Geometry check sheet. Reference: drawing and pictorial views, mm from the part's lowest x, y, z. A direction names the side the tool comes from. Round coordinates to 2 decimals unless told otherwise and drop trailing zeros. Write each loop counter-clockwise with the first axis right and the second up, starting at its lowest first coordinate (ties: lowest second). Pieces come first, ordered by that corner, then holes. Notation, with made-up numbers: (9, 29) -> (36, 29) arc R27 ccw to (36, 55) -> close; hole circle Ø3 at (39.25, 74.25). An arc over 180 degrees is marked (long way). Answer as a JSON object with one key per item and string values. Group by question number.
(1) Scan lines: L1, parallel to Y at x = 4.75, z = 5.25; L2, parallel to Y at x = 3.5, z = 4.25; L3, parallel to Z at x = 5, y = 6. Record each from-to range of solid material in increasing order. Write a range as from..to.
(2) Set-up check for the marked faces 1 and 2: record each of +Z, -Z, +X, -X, +Y, -Y from which the full face is reachable in a straight line by a thin tool's end or side.
(3) Gauge pin test, flat ends, axial feed: pin 1 Ø3 at (x, y) = (3, 2.5) entering from +Z; pin 2 Ø1 at (y, z) = (1, 1) entering from -X; pin 3 Ø0.7 at (x, z) = (5, 4) entering from -Y; pin 4 Ø4 at (y, z) = (4, 2) entering from +X. Record the tip position at first contact, or that the pin passes through.
(4) Sectioned sample at A-A on y = 4. Record the cut outline in (x, z).
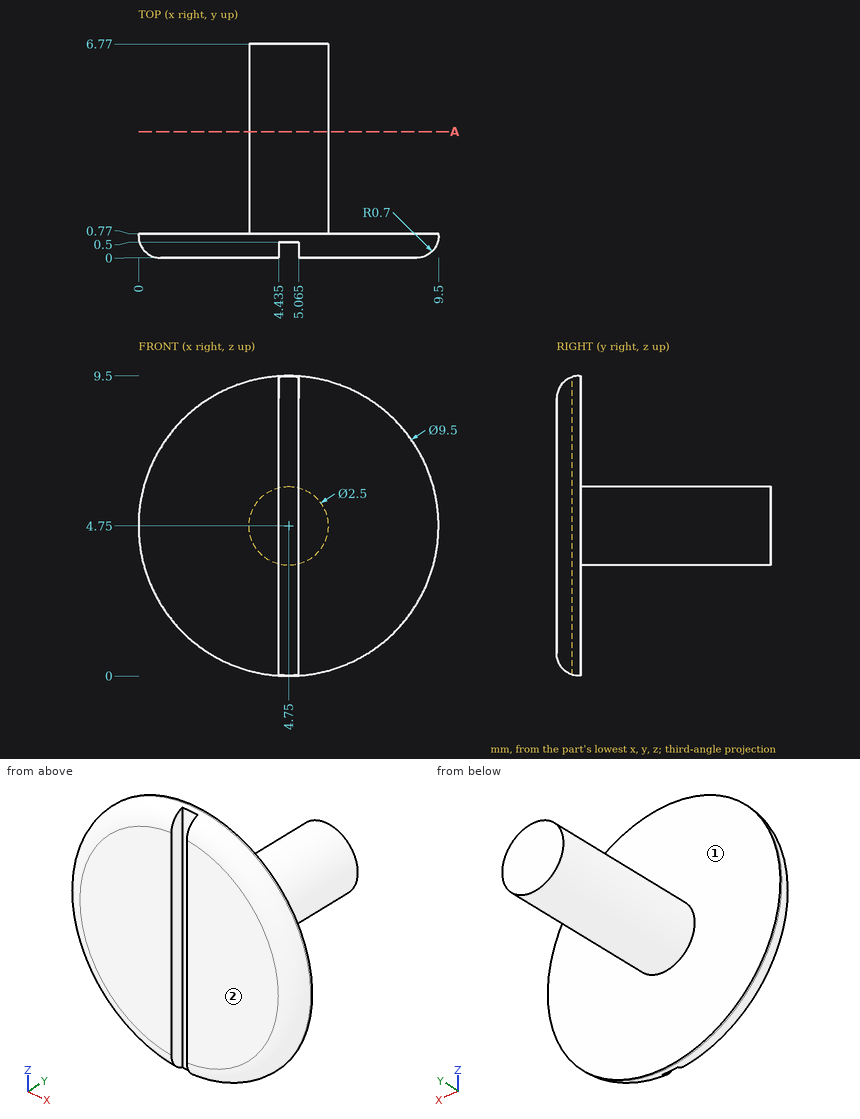
Computed values:
{
 "1": {"L1": "0.5..6.77", "L2": "0..0.77", "L3": "3.53..5.97"},
 "2": {"face 1": "+Y", "face 2": "+Z, -Z, +X, -X, -Y"},
 "3": {"pin 1": "z = 5.97", "pin 2": "x = 1.34", "pin 3": "y = 0", "pin 4": "x = 5.75"},
 "4": {"outline": "circle Ø2.5 at (4.75, 4.75)"}
}
